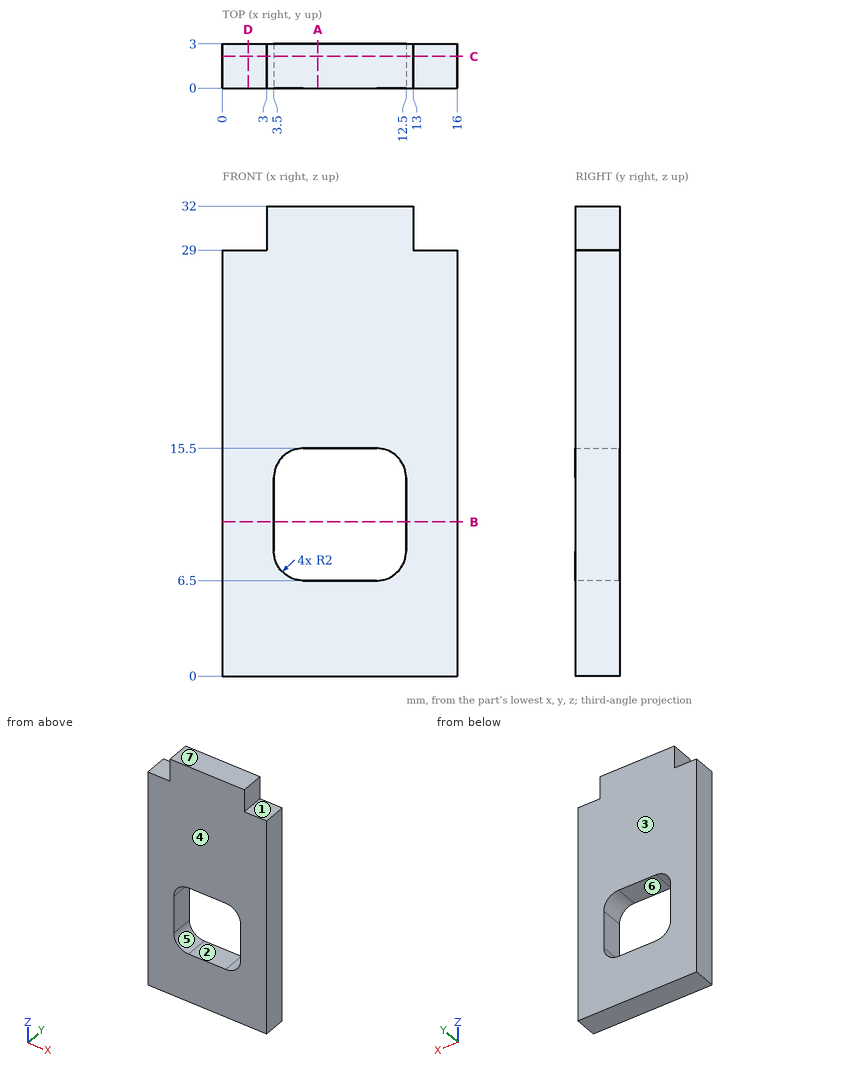
For this review, use the dimensioned drawing (mm, ordinates from the lowest corner) and the shaded views. A direction names the side the tool comes from. Round coordinates to 2 decimals unless told otherwise and drop trailing zeros. Order: outer loops, then holes, each group sorted by start corner. A loop starts at its lowest first (then second) coordinate and runs counter-clockwise, first axis right, second up.
1) Clearance check with flat-ended pins moving along their axes: pin 1 Ø1.5 at (x, z) = (11.5, 13.5) entering from +Y; pin 2 Ø0.9 at (x, y) = (1.5, 1.5) entering from +Z. State where each tip first meets the part, or that it passes through.
The answers:
pin 1: passes through
pin 2: stops at z = 29
2) Consider section B-B (z = 10.5). State the section outline as (x, y) points, plus the area to 3 significant figures.
The answers:
outline: (0, 0) - (3.5, 0) - (3.5, 3) - (0, 3) - close; (12.5, 0) - (16, 0) - (16, 3) - (12.5, 3) - close
area: 21.0 mm2
3) Consider section D-D (x = 1.75). State the section outline as (y, z) points.
The answers:
outline: (0, 0) - (3, 0) - (3, 29) - (0, 29) - close
4) Consider section A-A (x = 6.5). State the section outline as (y, z) points, plus the area to 3 significant figures.
The answers:
outline: (0, 0) - (3, 0) - (3, 6.5) - (0, 6.5) - close; (0, 15.5) - (3, 15.5) - (3, 32) - (0, 32) - close
area: 69.0 mm2
5) For L1, parallel to Z at x = 9.5, y = 1; L2, parallel to X at y = 1.8, z = 9.5; L3, parallel to X at y = 2, z = 30.5, list the stretches that pass through material, from the lowest coordinate up.
The answers:
L1: z = 0 to 6.5, 15.5 to 32
L2: x = 0 to 3.5, 12.5 to 16
L3: x = 3 to 13
6) Draft analysis for pull direction Z (two halves, no side actions). For the marked faces 4, 5, 6 and 7, state which applies: released by +Z, released by -Z, zero draft, split by the parting line, or undercut.
The answers:
face 4: zero draft
face 5: undercut
face 6: undercut
face 7: released by +Z
7) Machinability: for the marked faces 1, 2 and 3, which of the approach directions +Z, -Z, +X, -X, +Y, -Y give a long, thin tool a straight path to every point of the face, cutting with its end or side? Answer none if there is none.
The answers:
face 1: +Z, +X, +Y, -Y
face 2: +Y, -Y
face 3: +Z, -Z, +X, -X, +Y
8) Consider section C-C (y = 2.15). State the section outline as (x, z) points.
The answers:
outline: (0, 0) - (16, 0) - (16, 29) - (13, 29) - (13, 32) - (3, 32) - (3, 29) - (0, 29) - close; hole (3.5, 8.5) arc R2 ccw to (5.5, 6.5) - (10.5, 6.5) arc R2 ccw to (12.5, 8.5) - (12.5, 13.5) arc R2 ccw to (10.5, 15.5) - (5.5, 15.5) arc R2 ccw to (3.5, 13.5) - close
